```python
from build123d import *

# Parameters (mm, degrees)
SKETCH_1_R          = 8
EXTRUDE_1_DEPTH     = 2
SKETCH_3_R          = 1.1
SKETCH_3_R_2        = 1.75
CUT_EXTRUDE_1_DEPTH = 12.489125293


with BuildPart() as part:
    # 草图1 → 凸台-拉伸1 (new body)
    with BuildSketch(Plane.XY):
        Circle(SKETCH_1_R)
    extrude(amount=EXTRUDE_1_DEPTH)

    # 草图3 → 切除-拉伸1 (cut, through all)
    with BuildSketch(Plane(origin=(0, 0, 0), x_dir=(-1, 0, 0), z_dir=(0, 0, -1))):
        with Locations((0, 6)):
            Circle(SKETCH_3_R)
        with Locations((6, 0)):
            Circle(SKETCH_3_R)
        with Locations((0, -6)):
            Circle(SKETCH_3_R)
        with Locations((-6, 0)):
            Circle(SKETCH_3_R)
        Circle(SKETCH_3_R_2)
    extrude(amount=-CUT_EXTRUDE_1_DEPTH, mode=Mode.SUBTRACT)


solid = part.part
```
CAD build for the part. Positions are in the model's coordinates, mm. Round coordinates to 2 decimals unless told otherwise and drop trailing zeros. Order: outer loops, then holes, each group sorted by start corner. A loop starts at its lowest first (then second) coordinate and runs counter-clockwise, first axis right, second up.
Item 1: Mould opens along X. For faces 1 (the face through (0, 2, 2)), 2 (the face through (4.984, -0.421, 0.986)), 3 (the face through (-1.73, -7.81, 0.99)) say: pulls with the +X half, pulls with the -X half, needs draft (parallel to the pull), parting line crosses it, or undercut.
Item 2: Saw through at A-A on y = 0. Write the cut outline in (x, z), then the cut area to 3 significant figures.
Item 3: Probe line 1 along Y through (x, z) = (0, 1.4); line 2 along X through (y, z) = (-1, 0.65); line 3 along X through (y, z) = (1.25, 0.55). List the from-to ranges inside material, lowest first.
Item 4: Saw through at C-C on z = 0.8. Write the cut outline in (x, y), then the cut area to 3 significant figures.
Item 5: Pin check, flat tips, straight feed: pin 1 (2 mm diameter, centred on x = 0, y = 0, fed in from +Z); pin 2 (6 mm diameter, centred on x = 4.5, y = 5.5, fed in from -Z). Stop position of each tip, or through.
Item 6: Saw through at D-D on y = -6. Write the cut outline in (x, z).
Reported:
1. face 1: needs draft
1. face 2: undercut
1. face 3: parting line crosses it
2. outline: (-8, 0) - (-7.1, 0) - (-7.1, 2) - (-8, 2) - close; (-4.9, 0) - (-1.75, 0) - (-1.75, 2) - (-4.9, 2) - close; (1.75, 0) - (4.9, 0) - (4.9, 2) - (1.75, 2) - close; (7.1, 0) - (8, 0) - (8, 2) - (7.1, 2) - close
2. area: 16.2 mm2
3. line 1: y = -8 to -7.1, -4.9 to -1.75, 1.75 to 4.9, 7.1 to 8
3. line 2: x = -7.94 to -6.46, -5.54 to -1.44, 1.44 to 5.54, 6.46 to 7.94
3. line 3: x = -7.9 to -1.22, 1.22 to 7.9
4. outline: circle Ø16 at (0, 0); hole circle Ø2.2 at (-6, 0); hole circle Ø3.5 at (0, 0); hole circle Ø2.2 at (0, -6); hole circle Ø2.2 at (0, 6); hole circle Ø2.2 at (6, 0)
4. area: 176 mm2
5. pin 1: passes through
5. pin 2: stops at z = 0
6. outline: (-5.29, 0) - (-1.1, 0) - (-1.1, 2) - (-5.29, 2) - close; (1.1, 0) - (5.29, 0) - (5.29, 2) - (1.1, 2) - close
